from build123d import *

# Parameters (mm, degrees)
F0_R        = 2.4
F1_DEPTH    = 7.88
F2_T1_DEPTH = 26.405


# Not quite as in the source:
# - a fillet or chamfer that OpenCascade refuses, or shapes differently, is made with other operations: its cross-section is extruded or revolved along the edge and cut away or added


with BuildPart() as f1:
    # F0 (on Top) → F1 (new body)
    with BuildSketch(Plane.XY):
        Polygon((-14.7195083171, 1.6058013724), (-28.7195083171, 1.6058013724), (-42.7195083171, 1.6058013724), (-42.7195083171, -2.0891986276), (-42.7195083171, -5.7841986276), (-28.7195083171, -5.7841986276), (-14.7195083171, -5.7841986276), (-14.7195083171, -2.0891986276), align=None)
        with Locations((-36.7195083171, -2.0891986276)):
            Circle(F0_R, mode=Mode.SUBTRACT)
        with BuildLine():
            ThreePointArc((-28.7195083171, -4.4891986276), (-31.1195083171, -2.0891986276), (-28.7195083171, 0.3108013724))
            ThreePointArc((-28.7195083171, 0.3108013724), (-26.3195083171, -2.0891986276), (-28.7195083171, -4.4891986276))
        make_face(mode=Mode.SUBTRACT)
        with Locations((-20.7195083171, -2.0891986276)):
            Circle(F0_R, mode=Mode.SUBTRACT)
    extrude(amount=F1_DEPTH)

    # F2: fillet of radius 3.705 on 4 edges, made by hand

    # F2_s2 → F2_t1 (cut)
    with BuildSketch(Plane.XY.offset(-9.2625)):
        with BuildLine():
            ThreePointArc((-14.7195083171, -2.0991986276), (-15.8046776928, 0.5206319967), (-18.4245083171, 1.6058013724))
            Line((-18.4245083171, 1.6058013724), (-14.7195083171, 1.6058013724))
            Line((-14.7195083171, 1.6058013724), (-14.7195083171, -2.0991986276))
        make_face()
        with BuildLine():
            ThreePointArc((-14.7195083171, -2.0791986276), (-15.8046776928, -4.6990292519), (-18.4245083171, -5.7841986276))
            Line((-18.4245083171, -5.7841986276), (-14.7195083171, -5.7841986276))
            Line((-14.7195083171, -5.7841986276), (-14.7195083171, -2.0791986276))
        make_face()
        with BuildLine():
            ThreePointArc((-42.7195083171, -2.0991986276), (-41.6343389413, 0.5206319967), (-39.0145083171, 1.6058013724))
            Line((-39.0145083171, 1.6058013724), (-42.7195083171, 1.6058013724))
            Line((-42.7195083171, 1.6058013724), (-42.7195083171, -2.0991986276))
        make_face()
        with BuildLine():
            ThreePointArc((-42.7195083171, -2.0791986276), (-41.6343389413, -4.6990292519), (-39.0145083171, -5.7841986276))
            Line((-39.0145083171, -5.7841986276), (-42.7195083171, -5.7841986276))
            Line((-42.7195083171, -5.7841986276), (-42.7195083171, -2.0791986276))
        make_face()
    extrude(amount=F2_T1_DEPTH, mode=Mode.SUBTRACT)


solid = f1.part
The listing builds one solid part. Answer for the finished solid, in the listing's coordinates (mm). Round coordinates to 2 decimals unless told otherwise and drop trailing zeros. Write each loop counter-clockwise with the first axis right and the second up, starting at its lowest first coordinate (ties: lowest second). Pieces come first, ordered by that corner, then holes. Notation, with made-up numbers: (-10.5, -21) - (27.5, -21) arc R21 ccw to (27.5, 0) - close; hole circle Ø10 at (9.5, 1.25). An arc over 180 degrees is marked (long way). Use a Markdown table: item, result. Add a question column.
1. The part is cut by section A-A (y = -1.5). Write down the section's boundary in (x, z), and give its area (3 significant figures).
2. The part is cut by section C-C (z = 6.25). Write down the section's boundary in (x, y) (1 decimal), and give its area (3 significant figures).
3. The part is cut by section D-D (y = -3.75). Write down the section's boundary in (x, z).
4. A flat-ended cylindrical pin translates along its axis: P1, Ø2, axis at y = -4.5, z = 5.5, coming from the +X side. Find the tip coordinate at first contact, or state that the pin passes through.
5. Consider line 1 (X direction, y = -2.25, z = 1); line 2 (X direction, y = -1, z = 6.5); line 3 (Y direction, x = -38.75, z = 1.75). Determine where each line is inside the solid, lowest interval first.
6. The part is cut by section B-B (x = -38). Write down the section's boundary in (y, z), and give its area (3 significant figures).
7. For a pull along X with two mould halves and no side action, classify faces 1 (the face through (-15.78, 0.495, 3.885)), 2 (the face through (-23.117, -1.984, 3.885)), 3 (the face through (-29, 1.606, 4)) as +X half, -X half, draft (parallel to the pull), parting line (faces both ways), or undercut.
Reported:
| question | item | result |
|---|---|---|
| 1 | outline | (-42.67, 0) - (-39.05, 0) - (-39.05, 7.88) - (-42.67, 7.88) - close; (-34.39, 0) - (-31.05, 0) - (-31.05, 7.88) - (-34.39, 7.88) - close; (-26.39, 0) - (-23.05, 0) - (-23.05, 7.88) - (-26.39, 7.88) - close; (-18.39, 0) - (-14.77, 0) - (-14.77, 7.88) - (-18.39, 7.88) - close |
| 1 | area | 110 mm^2 |
| 2 | outline | (-42.7, -2.1) arc R3.7 ccw to (-39, -5.8) - (-18.4, -5.8) arc R3.7 ccw to (-14.7, -2.1) arc R3.7 ccw to (-18.4, 1.6) - (-39, 1.6) arc R3.7 ccw to start; hole circle Ø4.8 at (-36.7, -2.1); hole circle Ø4.8 at (-28.7, -2.1); hole circle Ø4.8 at (-20.7, -2.1) |
| 2 | area | 141 mm^2 |
| 3 | outline | (-42.32, 0) - (-38.45, 0) - (-38.45, 7.88) - (-42.32, 7.88) - close; (-34.99, 0) - (-30.45, 0) - (-30.45, 7.88) - (-34.99, 7.88) - close; (-26.99, 0) - (-22.45, 0) - (-22.45, 7.88) - (-26.99, 7.88) - close; (-18.99, 0) - (-15.12, 0) - (-15.12, 7.88) - (-18.99, 7.88) - close |
| 4 | P1 | x = -15 |
| 5 | line 1 | -42.72 to -39.11, -34.32 to -31.11, -26.32 to -23.11, -18.32 to -14.72 |
| 5 | line 2 | -42.55 to -38.86, -34.58 to -30.86, -26.58 to -22.86, -18.58 to -14.89 |
| 5 | line 3 | -5.78 to -3.37, -0.81 to 1.61 |
| 6 | outline | (-5.78, 0) - (-4.12, 0) - (-4.12, 7.88) - (-5.78, 7.88) - close; (-0.06, 0) - (1.61, 0) - (1.61, 7.88) - (-0.06, 7.88) - close |
| 6 | area | 26.2 mm^2 |
| 7 | face 1 | +X half |
| 7 | face 2 | undercut |
| 7 | face 3 | draft |
